Input: part model. Units: mm. Frame: model coordinates. A direction names the side the tool comes from. Give positions to 0.01 mm unless a question says otherwise; leave off trailing zeros. Loops run counter-clockwise (first coordinate to the right, second up) from the corner with the lowest first, then second, coordinate; pieces in that order, holes last.
from build123d import *

# Parameters (mm, degrees)
ESQUISSE1_R                  = 7
BOSS_EXTRU_1_DEPTH           = 8
ESQUISSE2_R                  = 7
ESQUISSE2_R_2                = 3
ENL_V_MAT_EXTRU_2_DEPTH      = 1.25
ENL_V_MAT_EXTRU_2_DEPTH_BACK = 1.25
CONG_1_R                     = 1
ENL_V_MAT_EXTRU_3_REACH      = 10
ESQUISSE3_R                  = 1.3


with BuildPart() as part:
    # Esquisse1 → Boss.-Extru.1 (new body)
    with BuildSketch(Plane.XY):
        Circle(ESQUISSE1_R)
    extrude(amount=BOSS_EXTRU_1_DEPTH)

    # Esquisse2 → Enlèv. mat.-Extru.2 (cut, two sides)
    with BuildSketch(Plane(origin=(0, 0, 4), x_dir=(-1, 0, 0), z_dir=(0, 0, -1))) as enl_v_mat_extru_2_sk:
        Circle(ESQUISSE2_R)
        Circle(ESQUISSE2_R_2, mode=Mode.SUBTRACT)
    extrude(amount=ENL_V_MAT_EXTRU_2_DEPTH, mode=Mode.SUBTRACT)
    extrude(enl_v_mat_extru_2_sk.sketch, amount=-ENL_V_MAT_EXTRU_2_DEPTH_BACK, mode=Mode.SUBTRACT)

    # Congé1
    cong_1_edges = [part.edges().sort_by_distance(p)[0] for p in [
        (3, 0, 2.75),
        (3, 0, 5.25),
    ]]
    fillet(cong_1_edges, radius=CONG_1_R)

    # Esquisse3 → Enlèv. mat.-Extru.3 (cut, up to next)
    with BuildSketch(Plane(origin=(0, 0, 0), x_dir=(-1, 0, 0), z_dir=(0, 0, -1)), mode=Mode.PRIVATE) as enl_v_mat_extru_3_sk1:
        Circle(ESQUISSE3_R)
    enl_v_mat_extru_3_tool1 = extrude(enl_v_mat_extru_3_sk1.sketch, amount=-ENL_V_MAT_EXTRU_3_REACH, mode=Mode.PRIVATE) & part.part
    add(enl_v_mat_extru_3_tool1.solids().sort_by_distance((0, 0, 0))[0], mode=Mode.SUBTRACT)


solid = part.part
(1) Ray query, probe 1 along Z at (x, y) = (5.5, 3); probe 2 along Y at (x, z) = (0, 6.25); probe 3 along Y at (x, z) = (0, 4). Return the intervals inside material, ascending.
Values follow:
probe 1: z = 0 to 2.75, 5.25 to 8
probe 2: y = -7 to -1.3, 1.3 to 7
probe 3: y = -3 to -1.3, 1.3 to 3
(2) Cut plane C-C (x = 5.5). Return the cut outline in (y, z), and give its area (3 significant figures).
Values follow:
outline: (-4.33, 0) - (4.33, 0) - (4.33, 2.75) - (-4.33, 2.75) - close; (-4.33, 5.25) - (4.33, 5.25) - (4.33, 8) - (-4.33, 8) - close
area: 47.6 mm2
(3) Pin query (flat end, axial travel): pin 1 Ø1.5 at (y, z) = (1, 5.5) entering from -X; pin 2 Ø2 at (x, z) = (3, 1) entering from +Y; pin 3 Ø1 at (x, z) = (1, 6) entering from -Y; pin 4 Ø1 at (x, z) = (-5.5, 4.5) entering from +Y. Return the tip coordinate at first contact, or that it passes through.
Values follow:
pin 1: stops at x = -7
pin 2: stops at y = 6.71
pin 3: stops at y = -6.98
pin 4: passes through
(4) Mould query, pull axis X, two halves, no side actions, for faces 1 (the cylindrical face through (6.466, -2.681, 1.356)), 2 (the flat face through (1.5, 0.1, 0)), 3 (the cylindrical face through (0.17, 1.29, 3.94)). Classes: +X half, -X half, draft (parallel to the pull), parting line (faces both ways), or undercut.
Values follow:
face 1: parting line
face 2: draft
face 3: undercut
(5) Cut plane A-A (y = 0). Return the cut outline in (x, z).
Values follow:
outline: (-7, 0) - (-1.3, 0) - (-1.3, 8) - (-7, 8) - (-7, 5.25) - (-4, 5.25) arc R1 cw to (-3, 4.25) - (-3, 3.75) arc R1 cw to (-4, 2.75) - (-7, 2.75) - close; (1.3, 0) - (7, 0) - (7, 2.75) - (4, 2.75) arc R1 cw to (3, 3.75) - (3, 4.25) arc R1 cw to (4, 5.25) - (7, 5.25) - (7, 8) - (1.3, 8) - close
(6) Cut plane D-D (z = 1.75). Return the cut outline in (x, y).
Values follow:
outline: circle Ø14 at (0, 0); hole circle Ø2.6 at (0, 0)
(7) Reachability of faces 4 (the cylindrical face through (6.466, -2.681, 6.606)), 5 (the flat face through (-3, -3, 5.25)) from +Z, -Z, +X, -X, +Y, -Y: full face, straight path, thin tool, end or side. Return the list, or none.
Values follow:
face 4: +Z, -Z
face 5: none
